```python
from build123d import *

# Parameters (mm, degrees)
F3_DEPTH      = 10.001
F3_DEPTH_BACK = 10.001
F4_R          = 0.5


with BuildPart() as f1:
    # F0 (on Right) → F1 (revolve)
    with BuildSketch(Plane.YZ):
        Polygon((-20, 3), (0, 3), (0, 10), (-40, 10), (-40, 7.5), (-20, 7.5), align=None)
    revolve(axis=Axis((0, -10.6568620467, 0), (0, -1, 0)))

    # F2 (on Top) → F3 (cut, two sides)
    with BuildSketch(Plane.XY) as f3_sk:
        with BuildLine():
            Line((-3, -30), (-3, -40))
            Line((-3, -40), (3, -40))
            Line((3, -40), (3, -30))
            ThreePointArc((3, -30), (0, -27), (-3, -30))
        make_face()
    extrude(amount=-F3_DEPTH, mode=Mode.SUBTRACT)
    extrude(f3_sk.sketch, amount=F3_DEPTH_BACK, mode=Mode.SUBTRACT)

    # F4
    f4_edges = [f1.edges().sort_by_distance(p)[0] for p in [
        (-3, -40, 8.206628),
        (-3, -40, -8.206628),
        (3, -40, 8.206628),
        (3, -40, -8.206628),
    ]]
    fillet(f4_edges, radius=F4_R)


solid = f1.part
```
The listing builds one solid part. Answer for the finished solid, in the listing's coordinates (mm). A direction names the side the tool comes from. Give positions to 0.01 mm unless a question says otherwise; leave off trailing zeros. Write each loop counter-clockwise with the first axis right and the second up, starting at its lowest first coordinate (ties: lowest second). Pieces come first, ordered by that corner, then holes. Notation, with made-up numbers: (53.5, 55) -> (64.5, 55) arc R18 cw to (64.5, 62) -> close; hole circle Ø7 at (28.5, 27). An arc over 180 degrees is marked (long way). Write item = value, one per line. Start each with the question number.
1) Each of these flat-tipped pins is pushed along its axis until it touches: pin 1 (5 mm diameter, centred on x = -7.5, y = -21.5, fed in from -Z); pin 2 (12 mm diameter, centred on x = -6, y = -35, fed in from +Z); pin 3 (2 mm diameter, centred on y = -35, z = -8, fed in from +X). Where does it stop, or does it pass through?
2) The part is cut by section B-B, the plane x = 0. Determine the outline of the cut face in (y, z).
3) Determine the mould class of faces 4 (the face through (-3, -20.28, 9.54)), 5 (the face through (-2.4, 0, -2.1)), 6 (the face through (4.564, -29.86, -5.952)) for opening direction Z: +Z half, -Z half, draft (parallel to the pull), parting line (faces both ways), or undercut.
4) The part is cut by section A-A, the plane z = 0. Determine the outline of the cut face in (x, y).
5) Which of the six approach directions +Z, -Z, +X, -X, +Y, -Y give full straight-line access (tool end or side, diameter ignored) to faces 1 (the face through (8, -40, 0)), 2 (the face through (3.2, -20, -0.1)), 3 (the face through (-3, -35, -8))?
6) Straight lines are drawn through the part: line 1 along Z through (x, y) = (0, -5.25); line 2 along X through (y, z) = (-25.25, 0). For each, find the intervals that lie inside material, in ascending order.
7) The part is cut by section C-C, the plane y = -19.5. Determine the outline of the cut face in (x, z).
8) The part is cut by section D-D, the plane x = -7. Determine the outline of the cut face in (y, z).
Solutions:
q1.pin_1 = -8.66
q1.pin_2 = 9.54
q1.pin_3 = 7.14
q2.outline = (-27, -10) -> (0, -10) -> (0, -3) -> (-20, -3) -> (-20, -7.5) -> (-27, -7.5) -> close; (-27, 7.5) -> (-20, 7.5) -> (-20, 3) -> (0, 3) -> (0, 10) -> (-27, 10) -> close
q3.face_4 = parting line
q3.face_5 = draft
q3.face_6 = undercut
q4.outline = (-10, -40) -> (-7.5, -40) -> (-7.5, -20) -> (-3, -20) -> (-3, 0) -> (-10, 0) -> close; (3, -20) -> (7.5, -20) -> (7.5, -40) -> (10, -40) -> (10, 0) -> (3, 0) -> close
q5.face_1 = +Z, -Z, +X, -X, -Y
q5.face_2 = -Y
q5.face_3 = +Z, -Z, -Y
q6.line_1 = -10 to -3, 3 to 10
q6.line_2 = -10 to -7.5, 7.5 to 10
q7.outline = circle Ø20 at (0, 0); hole circle Ø6 at (0, 0)
q8.outline = (-40, -7.14) -> (0, -7.14) -> (0, 7.14) -> (-40, 7.14) -> (-40, 2.69) -> (-20, 2.69) -> (-20, -2.69) -> (-40, -2.69) -> close
